Can you work these out from the model? Positions are in its coordinate system, mm. A direction names the side the tool comes from. Give positions to 0.01 mm unless a question says otherwise; leave off trailing zeros. Loops run counter-clockwise (first coordinate to the right, second up) from the corner with the lowest first, then second, coordinate; pieces in that order, holes last. Notation, with made-up numbers: (55, 37.5) -> (71, 37.5) arc R22 cw to (71, 61.5) -> close; hole circle Ø3 at (7.5, 13). An arc over 180 degrees is marked (long way). Return JSON: item names as keys, results as strings. Group by question number.
Q1. Suppose I cut it at A-A, the plane x = -54.5. Please give me the cut outline in (y, z).
Q2. I need wall thicknesses on line 1 along Z through (x, y) = (-3.5, 0.8); line 2 along Z through (x, y) = (-60.5, 0.5); line 3 along Z through (x, y) = (-24.5, 6.5). Which ranges of each line are inside material? Lowest first, please. Write a range as [from, to].
Q3. Suppose I cut it at D-D, the plane x = -30.5. Please give me the cut outline in (y, z).
Q4. Suppose I cut it at C-C, the plane y = 3.25. Please give me the cut outline in (x, z), and give its area (3 significant figures).
Q5. Thinking about a two-plate mould opening in Z: for faces 5 (the flat face through (-65, 5, -6.5)), 6 (the cylindrical face through (-59.36, 5.3, -24.4)), 7 (the flat face through (-65, 5, -23.5)), 8 (the flat face through (-12, 1.6, -31)), which applies, pulls with the +Z half, pulls with the -Z half, needs draft (parallel to the pull), parting line crosses it, or undercut?
Q6. Which directions (+Z, -Z, +X, -X, +Y, -Y) give clear straight access to the entire face, cutting with the end or side of a thin tool? Please do faces 1 (the flat face through (-12, 5.6, -30)), 2 (the flat face through (-54, 1.6, -31)), 3 (the cylindrical face through (-0.86, 0.79, -0.9)), 4 (the flat face through (-36.4, 4, -30)).
Q7. Suppose I cut it at B-B, the plane z = -18.5. Please give me the cut outline in (x, y), and give its area (4 significant figures).
Q8. Will these pins go through, and if not, where does the flat tip stop? pin 1 (2 mm diameter, centred on y = 3, z = -29, fed in from +X); pin 2 (2 mm diameter, centred on y = 4, z = -30, fed in from -X); pin 3 (1 mm diameter, centred on x = -57.5, y = 7, fed in from +Z).
Autodesk Inventor part; units mm, degrees
ref_plane "YZ Plane" through (0, 0, 0) normal (1, 0, 0) x (0, 1, 0)
ref_plane "XZ Plane" through (0, 0, 0) normal (0, 1, 0) x (-1, 0, 0)
ref_plane "XY Plane" through (0, 0, 0) normal (0, 0, 1) x (1, 0, 0)
sketch "Sketch1" plane through (0, 0, 0) normal (0, 1, 0) x (-1, 0, 0)
  line L0 (3, 0) -> (62, 0)
  line L1 (65, -3) -> (65, -27)
  line L2 (62, -30) -> (3, -30)
  line L3 (0, -27) -> (0, -3)
  arc A0 (65, -3) -> (62, 0) centre (62, -3) ccw
  arc A1 (62, -30) -> (65, -27) centre (62, -27) ccw
  arc A2 (0, -27) -> (3, -30) centre (3, -27) ccw
  arc A3 (3, 0) -> (0, -3) centre (3, -3) ccw
  circle A4 centre (61.5, -26.5) radius 1.25
  circle A5 centre (61.5, -3.5) radius 1.25
  circle A6 centre (3.5, -26.5) radius 1.25
  circle A7 centre (3.5, -3.5) radius 1.25
  point P0 (0, 0)
  point P1 (65, -30)
  point P2 (65, 0)
  point P3 (0, -30)
  dimension "d0" = 65
  dimension "d1" = 30
  dimension "d2" = 3
  dimension "d3" = 2.5
  dimension "d4" = 3.5
  dimension "d5" = 3.5
  dimension "d8" = 23
  dimension "d11" = 58
extrude "Extrusion1" add sketch "Sketch1" along normal blind 1.6
sketch "Sketch2" plane through (0, 1.6, 0) normal (0, 1, 0) x (1, 0, 0)
  circle A0 centre (-61.5, 26.5) radius 1.25
  line L0 (-65, 27) -> (-65, 3) construction
  line L1 (-65, 3) -> (-65, 27) construction
  line L2 (-3, 30) -> (-62, 30) construction
  line L3 (-62, 30) -> (-3, 30) construction
  circle A1 centre (-61.5, 26.5) radius 3 construction
  circle A2 centre (-61.5, 3.5) radius 3 construction
  circle A3 centre (-3.5, 26.5) radius 3 construction
  circle A4 centre (-3.5, 3.5) radius 3 construction
  circle A5 centre (-61.5, 3.5) radius 1.25 construction
  line L4 (-3.5, 3.5) -> (-61.5, 3.5) construction
  line L5 (-61.5, 3.5) -> (-61.5, 26.5) construction
  circle A6 centre (-3.5, 26.5) radius 1.25 construction
  line L6 (-61.5, 26.5) -> (-60.25, 26.5) construction
  circle A7 centre (-3.5, 3.5) radius 1.25 construction
  line L7 (-3.5, 26.5) -> (-3.5, 3.5) construction
  line L8 (-61.5, 3.5) -> (-61.5, 26.5) construction
  line L9 (-3.5, 26.5) -> (-61.5, 26.5) construction
  line L10 (-62, 0) -> (-3, 0) construction
  line L11 (-60.25, 26.5) -> (-3.5, 26.5) construction
  line L12 (-61.5, 6.5) -> (-61.5, 23.5)
  line L13 (-58.5, 26.5) -> (-6.5, 26.5)
  line L14 (-3.5, 23.5) -> (-3.5, 6.5)
  line L15 (-6.5, 3.5) -> (-58.5, 3.5)
  arc A8 (-61.5, 23.5) -> (-58.5, 26.5) centre (-61.5, 26.5) ccw
  arc A9 (-6.5, 26.5) -> (-3.5, 23.5) centre (-3.5, 26.5) ccw
  arc A10 (-3.5, 6.5) -> (-6.5, 3.5) centre (-3.5, 3.5) ccw
  arc A11 (-58.5, 3.5) -> (-61.5, 6.5) centre (-61.5, 3.5) ccw
  line L16 (-61.5, 6.5) -> (-68.5, 6.5)
  line L17 (-68.5, 6.5) -> (-68.5, 23.5)
  line L18 (-68.5, 23.5) -> (-61.5, 23.5)
  line L19 (-3.5, 6.5) -> (3.5, 6.5)
  line L20 (3.5, 6.5) -> (3.5, 23.5)
  line L21 (3.5, 23.5) -> (-3.5, 23.5)
  point P0 (0, 0)
  dimension "d17" = 6
  dimension "d20" = 23
  dimension "d23" = 58
  dimension "d28" = 7
  dimension "d29" = 7
extrude "Extrusion3" add sketch "Sketch2" along normal blind 7.5 contours L16 L17 L18 L12 | L12 A8 L13 A9 L14 A10 L15 A11
sketch "Sketch5" plane through (0, 1.6, 0) normal (0, 1, 0) x (1, 0, 0)
  line L0 (-6.5, 26.5) -> (-58.5, 26.5)
  line L1 (-36.4, 26.5) -> (-46.4, 26.5)
  line L2 (-46.4, 26.5) -> (-46.4, 32.5)
  line L3 (-46.4, 32.5) -> (-36.4, 32.5)
  line L4 (-36.4, 32.5) -> (-36.4, 26.5)
  line L5 (-41.4, 26.5) -> (-41.4, 32.5) construction
  line L6 (0, 3) -> (0, 27) construction
  line L7 (-49, 26.5) -> (-59, 26.5)
  line L8 (-59, 26.5) -> (-59, 32.5)
  line L9 (-59, 32.5) -> (-49, 32.5)
  line L10 (-49, 32.5) -> (-49, 26.5)
  line L11 (-54, 26.5) -> (-54, 32.5) construction
  line L12 (-58.5, 26.5) -> (-6.5, 26.5)
  line L13 (-6.4, 26.5) -> (-18.4, 26.5)
  line L14 (-18.4, 26.5) -> (-18.4, 32.5)
  line L15 (-18.4, 32.5) -> (-6.4, 32.5)
  line L16 (-6.4, 32.5) -> (-6.4, 26.5)
  line L17 (-12.4, 26.5) -> (-12.4, 32.5) construction
  point P0 (0, 0)
  dimension "d37" = 10
  dimension "d38" = 6
  dimension "d39" = 41.4
  dimension "d40" = 10
  dimension "d41" = 6
  dimension "d42" = 54
  dimension "d45" = 12
  dimension "d46" = 6
  dimension "d47" = 12.4
extrude "Extrusion5" add sketch "Sketch5" along normal blind 4
equation "\"d40\" = d37"
equation "\"d41\" = d38"
properties part number "RaspberryPi0W-SafeSpecs" material "ABS Plastic"
Ans:
{
 "1": {"outline": "(0, -30) -> (1.6, -30) -> (1.6, -32.5) -> (5.6, -32.5) -> (5.6, -26.5) -> (9.1, -26.5) -> (9.1, -3.5) -> (1.6, -3.5) -> (1.6, 0) -> (0, 0) -> close"},
 "2": {"line 1": "z = [-30, -27.75], [-25.25, -4.75], [-2.25, 0]", "line 2": "z = [-30, -27.25], [-25.75, -4.25], [-2.75, 0]", "line 3": "z = [-26.5, -3.5]"},
 "3": {"outline": "(0, -30) -> (1.6, -30) -> (1.6, -26.5) -> (9.1, -26.5) -> (9.1, -3.5) -> (1.6, -3.5) -> (1.6, 0) -> (0, 0) -> close"},
 "4": {"outline": "(-68.5, -23.5) -> (-61.5, -23.5) arc R3 cw to (-58.5, -26.5) -> (-59, -26.5) -> (-59, -32.5) -> (-49, -32.5) -> (-49, -26.5) -> (-46.4, -26.5) -> (-46.4, -32.5) -> (-36.4, -32.5) -> (-36.4, -26.5) -> (-18.4, -26.5) -> (-18.4, -32.5) -> (-6.4, -32.5) -> (-6.4, -26.5) -> (-6.5, -26.5) arc R3 cw to (-3.5, -23.5) -> (-3.5, -6.5) arc R3 cw to (-6.5, -3.5) -> (-58.5, -3.5) arc R3 cw to (-61.5, -6.5) -> (-68.5, -6.5) -> close", "area": "1,620 mm^2"},
 "5": {"face 5": "pulls with the +Z half", "face 6": "undercut", "face 7": "pulls with the -Z half", "face 8": "needs draft"},
 "6": {"face 1": "-Z, +X, -X, +Y", "face 2": "-Z, +X, -X, -Y", "face 3": "+Z, +X, +Y, -Y", "face 4": "-Z, +Y"},
 "7": {"outline": "(-68.5, 1.6) -> (-65, 1.6) -> (-65, 0) -> (0, 0) -> (0, 1.6) -> (-3.5, 1.6) -> (-3.5, 9.1) -> (-68.5, 9.1) -> close", "area": "591.5 mm^2"},
 "8": {"pin 1": "stops at x = -6.4", "pin 2": "stops at x = -59", "pin 3": "stops at z = -3.5"}
}
